from build123d import *

# Parameters (mm, degrees)
F0_W     = 25
F0_H     = 25
F1_DEPTH = 10
F2_R     = 5
F3_R     = 10.3297635793
F4_DEPTH = 9
F5_R     = 6.488280321
F6_DEPTH = 9
F8_D     = 3.3


with BuildPart() as f1:
    # F0 (on Front) → F1 (new body)
    with BuildSketch(Plane.XZ):
        Rectangle(F0_W, F0_H)
    extrude(amount=F1_DEPTH)

    # F2
    f2_edges = [f1.edges().sort_by_distance(p)[0] for p in [
        (12.5, -5, 12.5),
        (12.5, -5, -12.5),
        (-12.5, -5, 12.5),
        (-12.5, -5, -12.5),
    ]]
    fillet(f2_edges, radius=F2_R)

    # F3 (on face) → F4 (cut)
    with BuildSketch(Plane(origin=(0, 0, 0), x_dir=(-1, 0, 0), z_dir=(0, 1, 0))):
        Circle(F3_R)
    extrude(amount=-F4_DEPTH, mode=Mode.SUBTRACT)

    # F5 (on face) → F6 (join)
    with BuildSketch(Plane(origin=(0, -9, 0), x_dir=(-1, 0, 0), z_dir=(0, 1, 0))):
        Circle(F5_R)
    extrude(amount=F6_DEPTH)

    # F8 (through all)
    with Locations(Plane(origin=(0, 0, 0), x_dir=(-1, 0, 0), z_dir=(0, 1, 0))):
        with Locations((9.2421416193, 9.181400761), (9.181400761, -9.2421416193), (-9.2421416193, -9.181400761), (-9.181400761, 9.2421416193)):
            Hole(F8_D / 2)


solid = f1.part
Here's how the part is built. I have some questions about the finished solid (model axes, mm). A direction names the side the tool comes from. Give positions to 0.01 mm unless a question says otherwise; leave off trailing zeros. Order: outer loops, then holes, each group sorted by start corner. A loop starts at its lowest first (then second) coordinate and runs counter-clockwise, first axis right, second up. Notation, with made-up numbers: (31.5, -7.5) -> (52.5, -7.5) arc R24 ccw to (52.5, 25.5) -> close; hole circle Ø11 at (47.25, 65). An arc over 180 degrees is marked (long way). Use a Markdown table: item, result. Add a question column.
Item 1: Imagine slicing it at A-A on y = -0.75. Please give me the cut outline in (x, z).
Item 2: I need wall thicknesses on line 1 (Z direction, x = 2, y = -0.75); line 2 (X direction, y = -5, z = 1.25); line 3 (Z direction, x = 8.25, y = -0.5). Which ranges of each line are inside material? Lowest first, please.
Item 3: Imagine slicing it at C-C on x = 0. Please give me the cut outline in (y, z).
Item 4: Imagine slicing it at D-D on z = 0. Please give me the cut outline in (x, y).
Item 5: Imagine slicing it at B-B on z = 9.75. Please give me the cut outline in (x, y), plus the area to 3 significant figures.
Item 6: If we mould it in two halves opening along X, with no side actions, what happens to faces 1 (the face through (-10.458, -5.07, 10.297)), 2 (the face through (-7.5, 0, 7.5)), 3 (the face through (11, -5.07, -11.07))? For each: pulls with the +X half, pulls with the -X half, needs draft (parallel to the pull), parting line crosses it, or undercut.
Item 7: For faces 4 (the face through (0, -9, -7)), 5 (the face through (-11.07, -5.07, -11)), which set-ups out of +Z, -Z, +X, -X, +Y, -Y let a thin tool reach every point of the face, with its end or its side?
Item 8: Will this pin go through, and if not, where does the flat tip stop? pin 1 (10 mm diameter, centred on x = -1.5, z = 7.5, fed in from +Y).
Data:
| question | item | result |
|---|---|---|
| 1 | outline | (-12.5, -7.5) arc R5 ccw to (-7.5, -12.5) -> (7.5, -12.5) arc R5 ccw to (12.5, -7.5) -> (12.5, 7.5) arc R5 ccw to (7.5, 12.5) -> (-7.5, 12.5) arc R5 ccw to (-12.5, 7.5) -> close; circle Ø12.98 at (0, 0); hole circle Ø3.3 at (-9.24, 9.18); hole circle Ø3.3 at (-9.18, -9.24); hole circle Ø20.66 at (0, 0); hole circle Ø3.3 at (9.18, 9.24); hole circle Ø3.3 at (9.24, -9.18) |
| 2 | line 1 | z = -12.5 to -10.13, -6.17 to 6.17, 10.13 to 12.5 |
| 2 | line 2 | x = -12.5 to -10.25, -6.37 to 6.37, 10.25 to 12.5 |
| 2 | line 3 | z = -12.44 to -10.5, -7.86 to -6.22, 6.22 to 7.88, 10.6 to 12.44 |
| 3 | outline | (-10, -12.5) -> (0, -12.5) -> (0, -10.33) -> (-9, -10.33) -> (-9, -6.49) -> (0, -6.49) -> (0, 6.49) -> (-9, 6.49) -> (-9, 10.33) -> (0, 10.33) -> (0, 12.5) -> (-10, 12.5) -> close |
| 4 | outline | (-12.5, -10) -> (12.5, -10) -> (12.5, 0) -> (10.33, 0) -> (10.33, -9) -> (6.49, -9) -> (6.49, 0) -> (-6.49, 0) -> (-6.49, -9) -> (-10.33, -9) -> (-10.33, 0) -> (-12.5, 0) -> close |
| 5 | outline | (-11.97, -10) -> (-10.79, -10) -> (-10.79, 0) -> (-11.97, 0) -> close; (-7.69, -10) -> (7.61, -10) -> (7.61, 0) -> (3.41, 0) -> (3.41, -9) -> (-3.41, -9) -> (-3.41, 0) -> (-7.69, 0) -> close; (10.75, -10) -> (11.97, -10) -> (11.97, 0) -> (10.75, 0) -> close |
| 5 | area | 116 mm² |
| 6 | face 1 | undercut |
| 6 | face 2 | needs draft |
| 6 | face 3 | pulls with the +X half |
| 7 | face 4 | +Y |
| 7 | face 5 | -Z, -X, +Y, -Y |
| 8 | pin 1 | stops at y = 0 |
